Design review of the part built by this model. Coordinates are the model's own, in mm. Face numbers are marked on the shaded views. A direction names the side the tool comes from. Give positions to 0.01 mm unless a question says otherwise; leave off trailing zeros. Order: outer loops, then holes, each group sorted by start corner. A loop starts at its lowest first (then second) coordinate and runs counter-clockwise, first axis right, second up. Notation, with made-up numbers: (-26.75, 85) -> (25.25, 85) arc R32 ccw to (25.25, 118) -> close; hole circle Ø1 at (19, 5). An arc over 180 degrees is marked (long way). One line per item, written item: value. Start each with the question number.
1) Tool access review of the marked faces 1 and 2: name each direction out of +Z, -Z, +X, -X, +Y, -Y from which nothing blocks a thin tool from reaching the whole face with its end or side.
2) Consider section C-C (z = 2.3). State how many separate pieces and enclosed holes the cut face has, plus the area to 3 significant figures.
3) The part is to be moulded in two halves that separate along X. For the marked faces 3, 4 and 5, say which applies: released by +X, released by -X, zero draft, split by the parting line, or undercut.
4) Consider section B-B (y = -9). State the section outline as (x, z) points.
5) Consider section D-D (y = 19). State the section outline as (x, z) points.
6) For pin 1 (1.5 mm diameter, centred on x = 26.5, z = 3, fed in from -Y); pin 2 (2 mm diameter, centred on y = -1.5, z = 2, fed in from +X); pin 3 (2 mm diameter, centred on y = -1, z = 1.5, fed in from -X); pin 4 (5 mm diameter, centred on x = -14.09, y = -6.55, fed in from -Z), all flat-tipped, find the tip position at first contact; note any pin that passes through.
7) Wall thickness on line 1 along X through (y, z) = (-6.5, 3.5); line 2 along Y through (x, z) = (10, 0.35); line 3 along X through (y, z) = (-5, 1.15): over which ranges is each line inside the solid? List them lowest first. Write a range as from..to.
8) Consider section A-A (x = 8). State the section outline as (y, z) points, plus the area to 3 significant figures.
from build123d import *

# Parameters (mm, degrees)
BOSS_EXTRUDE1_DEPTH  = 4
FILLET1_R            = 8
FILLET2_R            = 2
SKETCH8_R            = 5
CUT_EXTRUDE1_DEPTH   = 4
SKETCH3_W            = 16
SKETCH3_H            = 8
BOSS_EXTRUDE2_DEPTH  = 4
SKETCH10_R           = 8
BOSS_EXTRUDE3_DEPTH  = 4
FILLET3_R            = 6
SKETCH11_R           = 4
CUT_EXTRUDE2_DEPTH   = 4
FILLET3_OF_MIRROR1_R = 6


with BuildPart() as part:
    # Sketch2 → Boss-Extrude1 (new body)
    with BuildSketch(Plane.XY):
        Polygon((-24.718317205, 0), (44.079761222, 0), (9.680722008, 38.594041061), align=None)
    extrude(amount=BOSS_EXTRUDE1_DEPTH)

    # Fillet1
    fillet1_edges = [part.edges().sort_by_distance(p)[0] for p in [
        (9.680722008, 38.594041061, 2),
    ]]
    fillet(fillet1_edges, radius=FILLET1_R)

    # Fillet2
    fillet2_edges = [part.edges().sort_by_distance(p)[0] for p in [
        (44.079761222, 0, 2),
        (-24.718317205, 0, 2),
    ]]
    fillet(fillet2_edges, radius=FILLET2_R)

    # Sketch8 → Cut-Extrude1 (cut)
    with BuildSketch(Plane.XY.offset(4)):
        with Locations((9.680722008, 22.887439188)):
            Circle(SKETCH8_R)
    extrude(amount=-CUT_EXTRUDE1_DEPTH, mode=Mode.SUBTRACT)

    # Sketch3 → Boss-Extrude2 (add)
    with BuildSketch(Plane.XY):
        with Locations((-14.081618267, -2.818082449)):
            Rectangle(SKETCH3_W, SKETCH3_H)
    boss_extrude2 = extrude(amount=BOSS_EXTRUDE2_DEPTH)

    # Sketch10 → Boss-Extrude3 (add)
    with BuildSketch(Plane.XY.offset(4)):
        with Locations((-14.092338513, -6.548407243)):
            Circle(SKETCH10_R)
    boss_extrude3 = extrude(amount=-BOSS_EXTRUDE3_DEPTH)

    # Fillet3
    fillet3_edges = [part.edges().sort_by_distance(p)[0] for p in [
        (-6.081618267, 0, 2),
    ]]
    fillet(fillet3_edges, radius=FILLET3_R)

    # Sketch11 → Cut-Extrude2 (cut)
    with BuildSketch(Plane.XY.offset(4)):
        with Locations((-14.092338513, -6.548407243)):
            Circle(SKETCH11_R)
    cut_extrude2 = extrude(amount=-CUT_EXTRUDE2_DEPTH, mode=Mode.SUBTRACT)

    # Mirror1: Boss-Extrude2, Boss-Extrude3, Cut-Extrude2 across plane
    add(boss_extrude2.mirror(Plane(origin=(9.7, 0, 0), x_dir=(0, 0, 1), z_dir=(1, 0, 0))))
    add(boss_extrude3.mirror(Plane(origin=(9.7, 0, 0), x_dir=(0, 0, 1), z_dir=(1, 0, 0))))
    add(cut_extrude2.mirror(Plane(origin=(9.7, 0, 0), x_dir=(0, 0, 1), z_dir=(1, 0, 0))), mode=Mode.SUBTRACT)

    # Fillet3 of Mirror1
    fillet3_of_mirror1_edges = [part.edges().sort_by_distance(p)[0] for p in [
        (25.481618267, 0, 2),
    ]]
    fillet(fillet3_of_mirror1_edges, radius=FILLET3_OF_MIRROR1_R)


solid = part.part
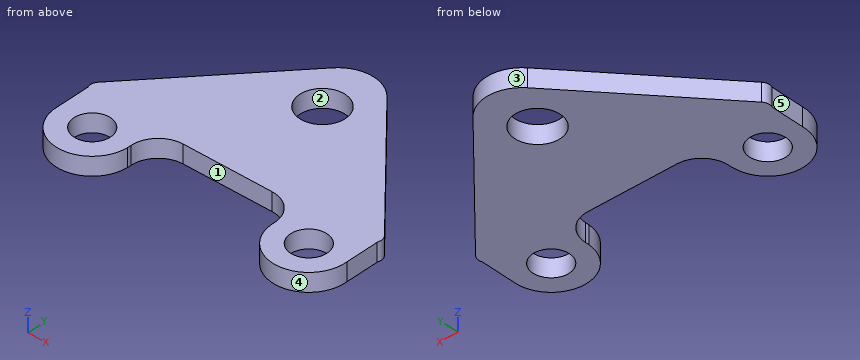
Checked values:
1. face 1: +Z, -Z, -Y
1. face 2: +Z, -Z
2. separate pieces: 1
2. enclosed holes: 3
2. area: 1,550 mm^2
3. face 3: split by the parting line
3. face 4: undercut
3. face 5: released by -X
4. outline: (-21.71, 0) -> (-17.25, 0) -> (-17.25, 4) -> (-21.71, 4) -> close; (-10.93, 0) -> (-6.48, 0) -> (-6.48, 4) -> (-10.93, 4) -> close; (25.88, 0) -> (30.33, 0) -> (30.33, 4) -> (25.88, 4) -> close; (36.65, 0) -> (41.11, 0) -> (41.11, 4) -> (36.65, 4) -> close
5. outline: (-7.78, 0) -> (6.54, 0) -> (6.54, 4) -> (-7.78, 4) -> close; (12.83, 0) -> (27.14, 0) -> (27.14, 4) -> (12.83, 4) -> close
6. pin 1: stops at y = -11.55
6. pin 2: stops at x = 41.48
6. pin 3: stops at x = -22.08
6. pin 4: passes through
7. line 1: x = -22.09..-18.09, -10.09..-6.08, 25.48..29.49, 37.49..41.49
7. line 2: y = 0..17.9, 27.88..34.56
7. line 3: x = -22.08..-17.78, -10.4..-6, 25.4..29.8, 37.18..41.48
8. outline: (0, 0) -> (18.18, 0) -> (18.18, 4) -> (0, 4) -> close; (27.6, 0) -> (34.39, 0) -> (34.39, 4) -> (27.6, 4) -> close
8. area: 99.9 mm^2
